Geometry check sheet. Reference: the model listing, model coordinates, mm. A direction names the side the tool comes from. Give positions to 0.01 mm unless a question says otherwise; leave off trailing zeros. Write each loop counter-clockwise with the first axis right and the second up, starting at its lowest first coordinate (ties: lowest second). Pieces come first, ordered by that corner, then holes.
(1) Tool access check on faces 5 (the flat face through (0, -432, -300)), 6 (the flat face through (-25.4, -432, -300)). Record the directions out of +Z, -Z, +X, -X, +Y, -Y that give a thin tool (end or side, any length) a straight path to the whole face; none if there is none.
(2) Depth check by flat-ended pin: P1, Ø4.5, axis at x = 24.63, y = -416.2, coming from the -Z side; P2, Ø8, axis at y = -352, z = -201.5, coming from the +X side. Enter the tip coordinate at first touch or a pass-through.
(3) Thickness scan on line 1 along Y through (x, z) = (217, -109.5); line 2 along Z through (x, y) = (258, -315.5); line 3 along X through (y, z) = (-413.5, -339). Record the ranges inside material, lowest first.
(4) Cross-section at C-C (y = -136.5). Record the boundary of the cut face in (x, z), and give its area (3 significant figures).
(5) Cross-section at A-A (x = 114.5). Record the boundary of the cut face in (y, z).
(6) Cross-section at B-B (z = -133). Record the boundary of the cut face in (x, y).
(7) Mould release check, pull along Z, two halves, no side actions. Record for faces 1 (the flat face through (137, 6.774, -300)), 2 (the flat face through (137, -432, 9.119)), 3 (the flat face through (137, -444, -600.481)), 4 (the flat face through (150, -856.826, -292)): +Z half, -Z half, draft (parallel to the pull), parting line (faces both ways), or undercut.
Autodesk Inventor part; units mm, degrees
ref_plane "YZ Plane" through (0, 0, 0) normal (1, 0, 0) x (0, 1, 0)
ref_plane "XZ Plane" through (0, 0, 0) normal (0, 1, 0) x (-1, 0, 0)
ref_plane "XY Plane" through (0, 0, 0) normal (0, 0, 1) x (1, 0, 0)
sketch "Sketch1" plane through (0, 0, 0) normal (1, 0, 0) x (0, 1, 0)
  line L0 (6.7738, 9.1186) -> (-882.2262, 9.1186)
  line L1 (-882.2262, 9.1186) -> (-882.2262, -600.4814)
  line L2 (-882.2262, -600.4814) -> (6.7738, -600.4814)
  line L3 (6.7738, -600.4814) -> (6.7738, 9.1186)
  line L4 (-18.6262, -16.2814) -> (-856.8262, -16.2814)
  line L5 (-856.8262, -16.2814) -> (-856.8262, -575.0814)
  line L6 (-856.8262, -575.0814) -> (-18.6262, -575.0814)
  line L7 (-18.6262, -575.0814) -> (-18.6262, -16.2814)
  point P0 (0, 0)
  dimension "d0" = 889
  dimension "d1" = 609.6
  dimension "d2" = 25.4
extrude "Extrusion3" add sketch "Sketch1" along normal blind 304.8
sketch "Sketch4" plane through (0, 0, 0) normal (-1, 0, 0) x (0, 0, 1)
  line L0 (9.1186, 6.7738) -> (9.1186, -882.2262)
  line L1 (9.1186, -882.2262) -> (-600.4814, -882.2262)
  line L2 (9.1186, 6.7738) -> (-600.4814, 6.7738)
  line L3 (-600.4814, 6.7738) -> (-600.4814, -882.2262)
  line L4 (-600.4814, -882.2262) -> (9.1186, -882.2262)
  line L5 (9.1186, -882.2262) -> (9.1186, 6.7738)
  point P0 (0, 0)
extrude "Extrusion4" add sketch "Sketch4" along normal blind 25.4
sketch "Sketch5" plane through (304.8, -882.2262, -600.4814) normal (0, 0, -1) x (-1, 0, 0)
  line L0 (0, 889) -> (330.2, 889)
  line L1 (330.2, 889) -> (330.2, 645.5901)
  line L2 (330.2, 889) -> (330.2, 0)
  line L3 (330.2, 457.2) -> (330.2, 279.4)
  line L4 (330.2, 279.4) -> (330.2, 101.6)
  line L5 (330.2, 518.5901) -> (609.6, 518.5901) construction
  line L6 (330.2, 340.7901) -> (609.6, 340.7901) construction
  line L7 (330.2, 162.9901) -> (609.6, 162.9901) construction
  line L8 (330.2, 457.2) -> (280.1718, 466.0213)
  line L9 (330.2, 457.2) -> (381, 457.2) construction
  line L10 (330.2, 279.4) -> (280.1718, 288.2213)
  line L11 (330.2, 279.4) -> (381, 279.4) construction
  line L12 (330.2, 101.6) -> (280.1718, 110.4213)
  line L13 (330.2, 101.6) -> (381, 101.6) construction
  line L14 (330.2, 0) -> (0, 0)
  line L15 (330.2, 0) -> (330.2, 101.6)
  circle A0 centre (280.1718, 466.0213) radius 2.5797
  circle A1 centre (280.1718, 288.2213) radius 2.5797
  circle A2 centre (280.1718, 110.4213) radius 2.5797
  line L16 (330.2, 457.2) -> (142.9418, 588.3196)
  line L17 (330.2, 457.2) -> (558.8, 457.2) construction
  line L18 (330.2, 279.4) -> (142.9418, 410.5196)
  line L19 (330.2, 279.4) -> (558.8, 279.4) construction
  line L20 (330.2, 101.6) -> (142.9418, 232.7196)
  line L21 (330.2, 101.6) -> (558.8, 101.6) construction
  circle A3 centre (142.9418, 588.3196) radius 2.5797
  circle A4 centre (142.9418, 410.5196) radius 2.5797
  circle A5 centre (142.9418, 232.7196) radius 2.5797
  point P0 (304.8, 882.2262)
  dimension "d16" = 177.8
  dimension "d17" = 177.8
  dimension "d35" = 50.8
  dimension "d36" = 170
  dimension "d37" = 50.8
  dimension "d38" = 170
  dimension "d39" = 50.8
  dimension "d40" = 170
  dimension "d46" = 101.6
  dimension "d48" = 5.1594
  dimension "d50" = 5.1594
  dimension "d52" = 5.1594
  dimension "d53" = 228.6
  dimension "d54" = 145
  dimension "d55" = 228.6
  dimension "d56" = 145
  dimension "d57" = 228.6
  dimension "d58" = 145
  dimension "d59" = 5.1594
  dimension "d60" = 5.1594
  dimension "d61" = 5.1594
extrude "Extrusion6" cut sketch "Sketch5" against normal blind 914.4
properties part number "Cart Box"
Reply:
1. face 5: +X
1. face 6: +Z, -Z, -X, +Y, -Y
2. P1: passes through
2. P2: stops at x = 0
3. line 1: y = -882.23 to -856.83, -18.63 to 6.77
3. line 2: z = -600.48 to -575.08, -16.28 to 9.12
3. line 3: x = -25.4 to 0
4. outline: (-25.4, -600.48) - (304.8, -600.48) - (304.8, -575.08) - (0, -575.08) - (0, -16.28) - (304.8, -16.28) - (304.8, 9.12) - (-25.4, 9.12) - close
4. area: 31,000 mm2
5. outline: (-882.23, -600.48) - (6.77, -600.48) - (6.77, 9.12) - (-882.23, 9.12) - close; hole (-856.83, -575.08) - (-18.63, -575.08) - (-18.63, -16.28) - (-856.83, -16.28) - close
6. outline: (-25.4, -882.23) - (304.8, -882.23) - (304.8, -856.83) - (0, -856.83) - (0, -18.63) - (304.8, -18.63) - (304.8, 6.77) - (-25.4, 6.77) - close
7. face 1: draft
7. face 2: +Z half
7. face 3: -Z half
7. face 4: undercut
